Work out the finished part from the listing and answer in its coordinate system (mm). Face numbers are marked on the shaded views. Coordinates: 2 decimals unless noted, no trailing zeros. Order: outer loops, then holes, each group sorted by start corner. A loop starts at its lowest first (then second) coordinate and runs counter-clockwise, first axis right, second up.
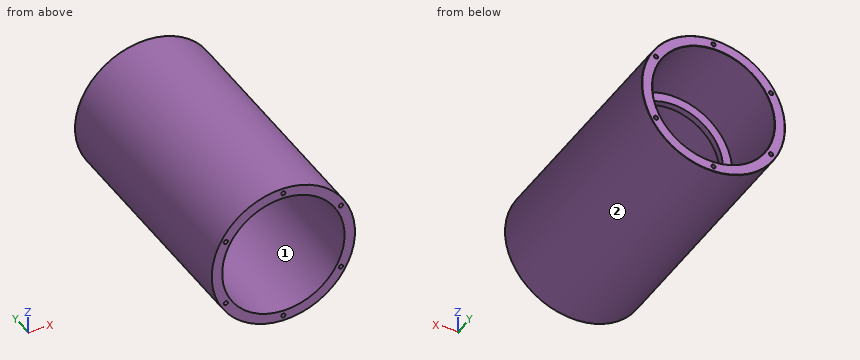
Autodesk Inventor part; units mm, degrees
ref_plane "YZ Plane" through (0, 0, 0) normal (1, 0, 0) x (0, 1, 0)
ref_plane "XZ Plane" through (0, 0, 0) normal (0, 1, 0) x (-1, 0, 0)
ref_plane "XY Plane" through (0, 0, 0) normal (0, 0, 1) x (1, 0, 0)
sketch "Skizze1" plane through (0, 0, 0) normal (1, 0, 0) x (0, 1, 0)
  line L0 (204.625, 55) -> (0, 55)
  line L1 (0, 55) -> (0, 47)
  line L2 (0, 47) -> (204.625, 47)
  line L3 (204.625, 47) -> (204.625, 55)
  line L4 (0, 47) -> (8, 47)
  line L5 (8, 47) -> (8, 0)
  line L6 (8, 0) -> (0, 0)
  line L7 (0, 0) -> (0, 47)
  line L8 (-40.925, 0) -> (245.55, 0)
  line L9 (0, -11) -> (0, 66)
  point P0 (0, 0)
  point P1 (4, 0)
  dimension "d0" = 8
  dimension "d1" = 8
  dimension "d2" = 204.625
  dimension "d3" = 47
  dimension "d4" = 0
  dimension "d5" = 0
revolve "Umdrehung1" add sketch "Skizze1" angle 360 about axis through (0, -10, 0) along (0, 1, 0)
sketch "Skizze2" plane through (0, 204.625, 0) normal (0, 1, 0) x (1, 0, 0)
  circle A0 centre (0, 0) radius 51 construction
  circle A1 centre (0, 0) radius 55
  circle A2 centre (0, 0) radius 51 construction
  circle A3 centre (0, 0) radius 51 construction
  circle A4 centre (0, 0) radius 51 construction
  circle A5 centre (0, 0) radius 51 construction
  circle A6 centre (0, 0) radius 51 construction
  point P0 (0, -51)
  point P1 (44.1673, -25.5)
  point P2 (44.1673, 25.5)
  point P3 (0, 51)
  point P4 (-44.1673, 25.5)
  point P5 (-44.1673, -25.5)
  dimension "d16" = 4
  dimension "d19" = 360
hole "Bohrung1" at (0, 204.625, 51) at (44.1673, 204.625, 25.5) at (44.1673, 204.625, -25.5) at (0, 204.625, -51) at (-44.1673, 204.625, -25.5) at (-44.1673, 204.625, 25.5) direction (0, -1, 0) diameter 3.242 depth 11.8 tip angle 118
chamfer "Fase1" distance 0.25 angle 45 1 edges at (0, 204.625, -47)
chamfer "Fase2" distance 0.25 angle 45 1 edges at (0, 204.625, -55)
chamfer "Fase3" distance 0.25 angle 45 1 edges at (0, 0, -55)
sketch "Skizze3" plane through (0, 0, 0) normal (0, -1, 0) x (1, 0, 0)
  circle A0 centre (0, 0) radius 60.1977
extrude "Extrusion1" cut sketch "Skizze3" against normal blind 10
ref_plane "Arbeitsebene1" through (0, 104.8125, 0) normal (0, 1, 0) x (1, 0, 0)
mirror "Spiegeln1" about plane through (0, 104.8125, 0) normal (0, 1, 0) of "Bohrung1"
ref_plane "Arbeitsebene3" through (0, 139.125, 0) normal (0, 1, 0) x (1, 0, 0)
sketch "Skizze4" plane through (0, 139.125, 0) normal (0, 1, 0) x (1, 0, 0)
  circle A0 centre (0, 0) radius 47
  circle A1 centre (0, 0) radius 47
  circle A2 centre (0, 0) radius 47
  circle A3 centre (0, 0) radius 47
  circle A4 centre (0, 0) radius 40
  dimension "d33" = 7
extrude "Extrusion2" add sketch "Skizze4" along normal blind 5
sketch "Skizze5" plane through (0, 204.625, 0) normal (0, 1, 0) x (1, 0, 0)
  point P0 (-44.1673, -25.5)
hole "Bohrung2" at (-44.1673, 204.625, 25.5) direction (0, -1, 0) diameter 3.242 depth 8 tip angle 120
properties part number "Gehäuse"
1. The part is cut by section A-A (z = 0). Determine the outline of the cut face in (x, y) (3 decimals), plus the area to 3 significant figures.
2. Consider probe 1 along Z at (x, y) = (1, 189.5); probe 2 along Z at (x, y) = (0, 142); probe 3 along Y at (x, z) = (-15.5, -38) (3 decimals). Determine where each line is inside the solid, lowest interval first.
3. The mould has two halves that part along X. Classify the marked faces 1 and 2: released by +X, released by -X, zero draft, split by the parting line, or undercut.
4. The part is cut by section B-B (y = 70.5). Determine the outline of the cut face in (x, z), plus the area to 3 significant figures.
5. Flat-ended cylindrical pins translate along their axes: pin 1 (10 mm diameter, centred on y = 57, z = -31.5, fed in from +X); pin 2 (6 mm diameter, centred on x = -14.5, y = 88, fed in from -Z); pin 3 (3 mm diameter, centred on x = -44.17, z = 25.5, fed in from +Y). Find the tip coordinate at first contact, or state that the pin passes through.
Worked out:
1. outline: (-55, 10) - (-47, 10) - (-47, 139.125) - (-40, 139.125) - (-40, 144.125) - (-47, 144.125) - (-47, 204.375) - (-47.25, 204.625) - (-54.75, 204.625) - (-55, 204.375) - close; (40, 139.125) - (47, 139.125) - (47, 10) - (55, 10) - (55, 204.375) - (54.75, 204.625) - (47.25, 204.625) - (47, 204.375) - (47, 144.125) - (40, 144.125) - close
1. area: 3,180 mm2
2. probe 1: z = -54.99 to -46.99, 46.99 to 54.99
2. probe 2: z = -55 to -40, 40 to 55
2. probe 3: y = 139.125 to 144.125
3. face 1: undercut
3. face 2: split by the parting line
4. outline: circle Ø110 at (0, 0); hole circle Ø94 at (0, 0)
4. area: 2,560 mm2
5. pin 1: stops at x = 48.19
5. pin 2: stops at z = -53.78
5. pin 3: stops at y = 192.75
